Autodesk Inventor part; units mm, degrees
ref_plane "YZ Plane" through (0, 0, 0) normal (1, 0, 0) x (0, 1, 0)
ref_plane "XZ Plane" through (0, 0, 0) normal (0, 1, 0) x (-1, 0, 0)
ref_plane "XY Plane" through (0, 0, 0) normal (0, 0, 1) x (1, 0, 0)
sketch "Sketch1" plane through (0, 0, 0) normal (0, 1, 0) x (-1, 0, 0)
  circle A0 centre (0, 0) radius 12
  dimension "d0" = 24
extrude "Extrusion1" add sketch "Sketch1" along normal blind 100
sketch "Sketch2" plane through (0, 100, 0) normal (0, 1, 0) x (1, 0, 0)
  circle A0 centre (0, 0) radius 20
  dimension "d3" = 40
extrude "Extrusion2" add sketch "Sketch2" along normal blind 24
chamfer "Chamfer1" distance 8 angle 45 1 edges at (-20, 124, 0)
properties part number "axle"
Could you check a few things on this model? Use its own coordinates, in mm. A direction names the side the tool comes from. Coordinates: 2 decimals unless noted, no trailing zeros. Write each loop counter-clockwise with the first axis right and the second up, starting at its lowest first coordinate (ties: lowest second). Pieces come first, ordered by that corner, then holes. Notation, with made-up numbers: M -35,85.25 L 13,85.25 A24 cw 13,117.25 Z; hole C 18.5,-40 d6. An arc over 180 degrees is marked long. Answer as CSV lines item,"result". Start each with the question number.
1) Please list where these lines run through material, in increasing order: line 1 (Z direction, x = 0, y = 61); line 2 (Z direction, x = -1, y = 111.5); line 3 (X direction, y = 72.5, z = 4). Write a range as from..to.
2) For P1, Ø12, axis at y = 67.5, z = 2, coming from the +X side; P2, Ø1.5, axis at x = -10, y = 18, coming from the +Z side; P3, Ø5, axis at y = 40.5, z = 4.5, coming from the -X side, each with a flat end and sliding along its axis, tell me the tip position at first contact or that it passes through.
3) I want a section at B-B, the plane x = 0. Please give me the cut outline in (y, z), and give its area (3 significant figures).
4) I want a section at C-C, the plane y = 80. Please give me the cut outline in (x, z).
5) For faces 1 (the cylindrical face through (-4.336, 107.888, -19.524)), 2 (the cylindrical face through (11.99, 49.3, -0.53)), which set-ups out of +Z, -Z, +X, -X, +Y, -Y let a thin tool reach every point of the face, with its end or its side?
6) I want a section at A-A, the plane z = 0. Please give me the cut outline in (x, y), and give its area (3 significant figures).
Data:
1,line 1,"z = -12..12"
1,line 2,"z = -19.97..19.97"
1,line 3,"x = -11.31..11.31"
2,P1,"stops at x = 12"
2,P2,"stops at z = 7.64"
2,P3,"stops at x = -11.83"
3,outline,"M 0,-12 L 100,-12 L 100,-20 L 116,-20 L 124,-12 L 124,12 L 116,20 L 100,20 L 100,12 L 0,12 Z"
3,area,"3,300 mm^2"
4,outline,"C 0,0 d24"
5,face 1,"+Y, -Y"
5,face 2,"-Y"
6,outline,"M -20,100 L -12,100 L -12,0 L 12,0 L 12,100 L 20,100 L 20,116 L 12,124 L -12,124 L -20,116 Z"
6,area,"3,300 mm^2"
